Part model, mm, in its own coordinate system. Give positions to 0.01 mm unless a question says otherwise; leave off trailing zeros. Write each loop counter-clockwise with the first axis right and the second up, starting at its lowest first coordinate (ties: lowest second). Pieces come first, ordered by that corner, then holes. Notation, with made-up numbers: (-31, -33) - (-22, -33) arc R28 ccw to (-22, -14) - close; hole circle Ø8 at (33.25, -10). An arc over 180 degrees is marked (long way). Answer in a Markdown table with one row per item. Add a question column.
1. Band-saw the part on C-C on y = 6. Write the cut outline in (x, z).
2. Probe line 1 along Z through (x, y) = (-16, 4.25); line 2 along Y through (x, z) = (4, -18); line 3 along Z through (x, y) = (7.5, 1.1). List the from-to ranges inside material, lowest first.
3. Drop flat-ended pins along their axis: pin 1 Ø4 at (x, z) = (-7, 12) entering from +Y; pin 2 Ø3 at (y, z) = (6, 11) entering from -X; pin 3 Ø5 at (x, z) = (-19.5, 17) entering from +Y. Give the stop position or say it passes through.
4. Band-saw the part on A-A on z = 0. Write the cut outline in (x, y) (3 decimals), plus the area to 3 significant figures.
5. Band-saw the part on B-B on x = 0. Write the cut outline in (y, z).
6. Band-saw the part on D-D on y = 1.5. Write the cut outline in (x, z) (3 decimals), plus the area to 3 significant figures.
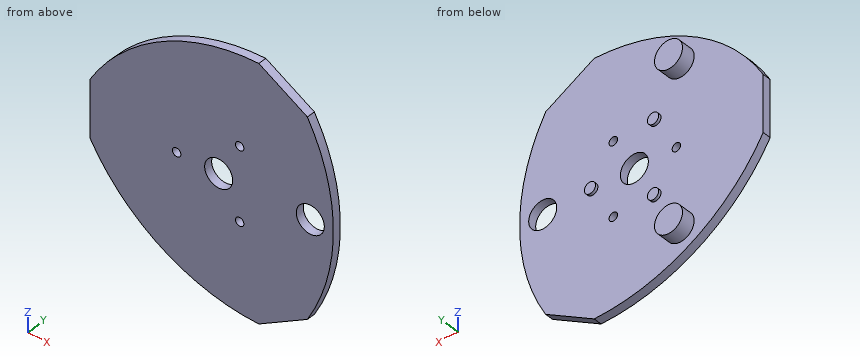
Autodesk Inventor part; units mm, degrees
ref_plane "YZ Plane" through (0, 0, 0) normal (1, 0, 0) x (0, 1, 0)
ref_plane "XZ Plane" through (0, 0, 0) normal (0, 1, 0) x (-1, 0, 0)
ref_plane "XY Plane" through (0, 0, 0) normal (0, 0, 1) x (1, 0, 0)
sketch "Sketch1" plane through (0, 0, 0) normal (0, 1, 0) x (-1, 0, 0)
  circle A0 centre (0, 0) radius 25
  circle A1 centre (0, 0) radius 5
  circle A2 centre (15, 0) radius 1.505
  line L0 (46, 0) -> (46, -10)
  line L1 (46, -10) -> (40, -10)
  line L2 (34, 0) -> (34, -10)
  line L3 (34, -10) -> (40, -10)
  line L4 (34, 0) -> (46, 0)
  line L5 (46, 0) -> (46, 10)
  line L6 (46, 10) -> (34, 10)
  line L7 (34, 10) -> (34, 0)
  line L8 (-23, 39.8372) -> (-14.3397, 44.8372)
  line L9 (-14.3397, 44.8372) -> (-11.3397, 39.641)
  line L10 (-17, 29.4449) -> (-8.3397, 34.4449)
  line L11 (-8.3397, 34.4449) -> (-11.3397, 39.641)
  line L12 (-17, 29.4449) -> (-23, 39.8372)
  line L13 (-23, 39.8372) -> (-31.6603, 34.8372)
  line L14 (-31.6603, 34.8372) -> (-25.6603, 24.4449)
  line L15 (-25.6603, 24.4449) -> (-17, 29.4449)
  line L16 (-23, -39.8372) -> (-31.6603, -34.8372)
  line L17 (-31.6603, -34.8372) -> (-28.6603, -29.641)
  line L18 (-17, -29.4449) -> (-25.6603, -24.4449)
  line L19 (-25.6603, -24.4449) -> (-28.6603, -29.641)
  line L20 (-17, -29.4449) -> (-23, -39.8372)
  line L21 (-23, -39.8372) -> (-14.3397, -44.8372)
  line L22 (-14.3397, -44.8372) -> (-8.3397, -34.4449)
  line L23 (-8.3397, -34.4449) -> (-17, -29.4449)
  circle A3 centre (-7.5, 12.9904) radius 1.505
  circle A4 centre (-7.5, -12.9904) radius 1.505
  circle A5 centre (-15, 0) radius 2.005
  circle A6 centre (7.5, -12.9904) radius 2.005
  circle A7 centre (7.5, 12.9904) radius 2.005
  arc A8 (46, 10) -> (-14.3397, 44.8372) centre (-14.5276, -25.1626) ccw
  arc A9 (-14.3397, -44.8372) -> (46, -10) centre (-14.5276, 25.1626) ccw
  arc A10 (-31.6603, 34.8372) -> (-31.6603, -34.8372) centre (29.0552, 0) ccw
  point P0 (40, 0)
  dimension "d22" = 360
  dimension "d26" = 360
  dimension "d32" = 360
  dimension "d34" = 70
  dimension "d35" = 70
  dimension "d36" = 70
  dimension "d90" = 10
extrude "Extrusion1" add sketch "Sketch1" along normal blind 3 contours L0 L1 L3 L2 L4 | L4 L7 L6 L5 | A9 L22 L23 L18 L19 L17 A10 L14 L15 L10 L11 L9 A8 L6 L7 L2 L3 L1 | L21 L20 L23 L22 | L9 L11 L10 L12 L8 | L16 L17 L19 L18 L20 | L12 L15 L14 L13
sketch "Sketch2" plane through (0, 3, 0) normal (0, 1, 0) x (1, 0, 0)
  circle A0 centre (32.7082, 0) radius 5
  circle A1 centre (-16.3541, 28.3261) radius 5
  circle A2 centre (-16.3541, -28.3261) radius 5
  point P0 (0, 0)
  dimension "d43" = 10
  dimension "d46" = 360
extrude "Extrusion4" add sketch "Sketch2" along normal blind 5 contours A1 | A2
extrude "Extrusion7" add sketch "Sketch1" along normal blind 3 contours A0
sketch "Sketch8" plane through (0, 3, 0) normal (0, 1, 0) x (1, 0, 0)
  point P0 (0, 0)
extrude "Extrusion9" add sketch "Sketch1" along normal blind 4 contours A5 | A6 | A7
extrude "Extrusion10" cut sketch "Sketch2" against normal blind 5 contours A0
equation "\"BendRadius\" = Thickness"
equation "\"BendReliefWidth\" = Thickness"
equation "\"BendReliefDepth\" = 0.5 * Thickness"
equation "\"CornerReliefSize\" = 4 * Thickness"
equation "\"MinimumRemnant\" = 2 * Thickness"
equation "\"TransitionRadius\" = BendRadius"
equation "\"JacobiRadiusSize\" = BendRadius"
equation "\"GapSize\" = Thickness"
properties part number "Tool_1"
Values:
| question | item | result |
|---|---|---|
| 1 | outline | circle Ø10 at (-16.35, -28.33); circle Ø10 at (-16.35, 28.33) |
| 2 | line 1 | z = -33.31 to -23.34, 23.34 to 33.31 |
| 2 | line 2 | y = 0 to 3 |
| 2 | line 3 | z = -44.48 to -14.5, -11.49 to 11.49, 14.5 to 44.48 |
| 3 | pin 1 | stops at y = 4 |
| 3 | pin 2 | passes through |
| 3 | pin 3 | stops at y = 3 |
| 4 | outline | (-46, 0) - (-16.505, 0) - (-16.505, 3) - (-46, 3) - close; (-13.495, 0) - (-5, 0) - (-5, 3) - (-13.495, 3) - close; (5, 0) - (27.708, 0) - (27.708, 3) - (17.005, 3) - (17.005, 4) - (12.995, 4) - (12.995, 3) - (5, 3) - close; (37.708, 0) - (40.945, 0) - (40.945, 3) - (37.708, 3) - close |
| 4 | area | 196 mm² |
| 5 | outline | (0, -43.31) - (3, -43.31) - (3, -5) - (0, -5) - close; (0, 5) - (3, 5) - (3, 43.31) - (0, 43.31) - close |
| 6 | outline | (-46, -10) arc R70 ccw to (14.34, -44.837) - (31.66, -34.837) arc R70 ccw to (31.66, 34.837) - (14.34, 44.837) arc R70 ccw to (-46, 10) - close; hole circle Ø3.01 at (-15, 0); hole circle Ø10 at (0, 0); hole circle Ø3.01 at (7.5, -12.99); hole circle Ø3.01 at (7.5, 12.99); hole circle Ø10 at (32.708, 0) |
| 6 | area | 5,820 mm² |
